```python
from build123d import *


with BuildPart() as f2:
    # F2: sweep along a path in F1
    with BuildLine(Plane.XY) as f2_path:
        Line((0, 0), (0, -89.280188))
        ThreePointArc((0, -89.280188), (-1.749391, -99.374895), (-6.793541, -108.292296))
        Line((-6.793541, -108.292296), (-75.132394, -191.707704))
        ThreePointArc((-75.132394, -191.707704), (-80.176544, -200.625105), (-81.925935, -210.719812))
        Line((-81.925935, -210.719812), (-81.925935, -550))
        Line((-81.925935, -550), (-81.925935, -889.280188))
        ThreePointArc((-81.925935, -889.280188), (-80.176544, -899.374895), (-75.132394, -908.292296))
        Line((-75.132394, -908.292296), (-6.793541, -991.707704))
        ThreePointArc((-6.793541, -991.707704), (-1.749391, -1000.625105), (0, -1010.719812))
        Line((0, -1010.719812), (0, -1100))
    # F0 (on Front) → F2 (sweep)
    with BuildSketch(Plane.XZ):
        with BuildLine():
            Line((10, 20), (-8, 20))
            ThreePointArc((-8, 20), (-9.414214, 19.414214), (-10, 18))
            Line((-10, 18), (-10, 17))
            ThreePointArc((-10, 17), (-9.414214, 15.585786), (-8, 15))
            Line((-8, 15), (-6, 15))
            ThreePointArc((-6, 15), (-4.585786, 14.414214), (-4, 13))
            Line((-4, 13), (-4, -13))
            ThreePointArc((-4, -13), (-4.585786, -14.414214), (-6, -15))
            Line((-6, -15), (-8, -15))
            ThreePointArc((-8, -15), (-9.414214, -15.585786), (-10, -17))
            Line((-10, -17), (-10, -18))
            ThreePointArc((-10, -18), (-9.414214, -19.414214), (-8, -20))
            Line((-8, -20), (10, -20))
            Line((10, -20), (10, 20))
        make_face()
    sweep(path=f2_path.line)


solid = f2.part
```
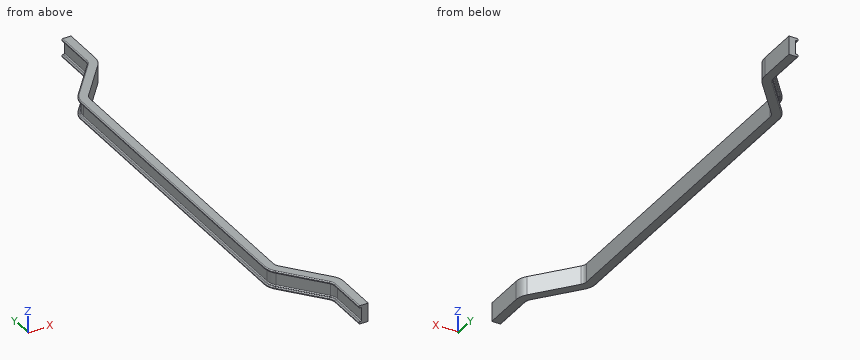
Geometry: final body of the model. Coordinates: model frame, mm. Give positions to 0.01 mm unless a question says otherwise; leave off trailing zeros. Loops run counter-clockwise (first coordinate to the right, second up) from the corner with the lowest first, then second, coordinate; pieces in that order, holes last. Notation, with made-up numbers: (-10.75, 76.5) - (47.25, 76.5) arc R29 cw to (47.25, 97.5) - close; hole circle Ø9 at (14.25, 14). An arc over 180 degrees is marked (long way). Answer as CSV lines item,"result". Start each with the question number.
(1) Pin query (flat end, axial travel): P1, Ø0.8, axis at y = -66, z = -17.5, coming from the -X side; P2, Ø8, axis at y = -698, z = 1.5, coming from the -X side; P3, Ø1.5, axis at x = -77, z = -10, coming from the +Y side. Return the tip coordinate at first contact, or that it passes through.
(2) Section query B-B (y = -499). Output: boundary loops of the cut face in (x, z).
(3) Ray query, line 1 along Z through (x, y) = (-88, -730); line 2 along X through (y, z) = (-802.5, 12); line 3 along Y through (x, z) = (-41, 1). Return the intervals inside material, ascending. Write a range as [from, to].
(4) Section query A-A (z = -1). Output: boundary loops of the cut face in (x, y), and give its area (3 significant figures).
Worked answers:
1,P1,"stops at x = -10"
1,P2,"stops at x = -85.93"
1,P3,"stops at y = -186.76"
2,outline,"(-91.93, -18) arc R2 ccw to (-89.93, -20) - (-71.93, -20) - (-71.93, 20) - (-89.93, 20) arc R2 ccw to (-91.93, 18) - (-91.93, 17) arc R2 ccw to (-89.93, 15) - (-87.93, 15) arc R2 cw to (-85.93, 13) - (-85.93, -13) arc R2 cw to (-87.93, -15) - (-89.93, -15) arc R2 ccw to (-91.93, -17) - close"
3,line 1,"z = [-20, -15], [15, 20]"
3,line 2,"x = [-85.93, -71.93]"
3,line 3,"y = [-956.27, -934.18], [-165.82, -143.73]"
4,outline,"(-85.93, -889.28) arc R34 ccw to (-78.23, -910.83) - (-9.89, -994.24) arc R26 cw to (-4, -1010.72) - (-4, -1100) - (10, -1100) - (10, -1010.72) arc R40 ccw to (0.94, -985.37) - (-67.4, -901.95) arc R20 cw to (-71.93, -889.28) - (-71.93, -210.72) arc R20 cw to (-67.4, -198.05) - (0.94, -114.63) arc R40 ccw to (10, -89.28) - (10, 0) - (-4, 0) - (-4, -89.28) arc R26 cw to (-9.89, -105.76) - (-78.23, -189.17) arc R34 ccw to (-85.93, -210.72) - close"
4,area,"16,200 mm^2"
